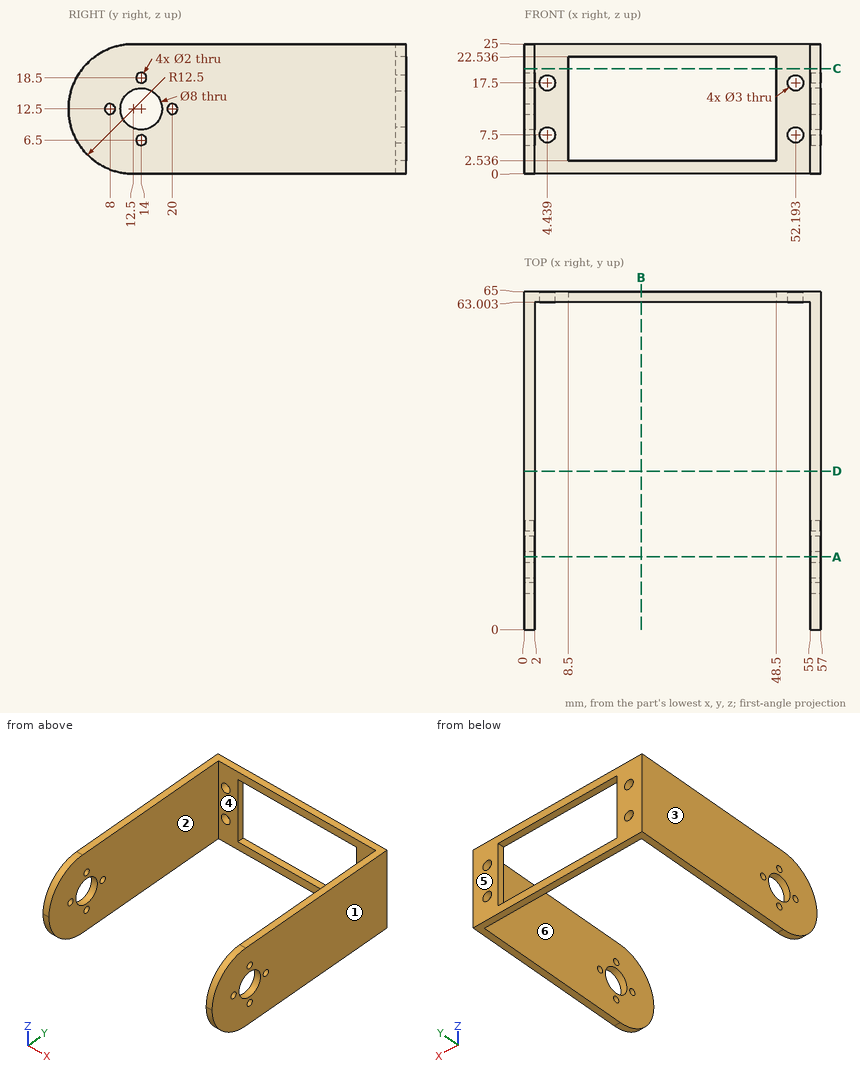
Drawing for the job (mm, zero at the part's lowest x, y, z). A direction names the side the tool comes from. Give positions to 0.01 mm unless a question says otherwise; leave off trailing zeros. Order: outer loops, then holes, each group sorted by start corner. A loop starts at its lowest first (then second) coordinate and runs counter-clockwise, first axis right, second up. Notation, with made-up numbers: M 59,29.25 L 70,29.25 A16 cw 70,41.25 Z; hole C 38.25,-37 d6. An arc over 180 degrees is marked long. Write item = value, one per line. Start each with the question number.
(1) Slice it at C-C on z = 20.25. Write the cut outline in (x, y), plus the area to 3 significant figures.
(2) Probe L1, parallel to X at y = 63.8, z = 17.5; L2, parallel to Z at x = 1.55, y = 14; L3, parallel to X at y = 36, z = 9.75. List the from-to ranges inside material, lowest first. Write a range as [from, to].
(3) Slice it at A-A on y = 14. State how many separate pieces and enclosed holes the cut face has.
(4) Slice it at D-D on y = 30.5. Write the cut outline in (x, z), plus the area to 3 significant figures.
(5) Slice it at B-B on x = 22.5. Write the cut outline in (y, z) (1 decimal).
(6) Two-plate mould, pull along X, no slides. Class the marked faces 3, 4, 5 and 6: released by +X, released by -X, zero draft, split by the parting line, or undercut.
(7) Which spindle directions (+Z, -Z, +X, -X, +Y, -Y) get a long thin tool onto all of the face, cutting with end or side? Do the marked faces 1 and 2. Say none if no direction does.
Responses:
q1.outline = M 0,2.69 L 2,2.69 L 2,63 L 8.5,63 L 8.5,65 L 0,65 Z; M 48.5,63 L 55,63 L 55,2.69 L 57,2.69 L 57,65 L 48.5,65 Z
q1.area = 275 mm2
q2.L1 = [0, 2.94], [5.94, 8.5], [48.5, 50.69], [53.69, 57]
q2.L2 = [0, 5.5], [7.5, 8.5], [16.5, 17.5], [19.5, 25]
q2.L3 = [0, 2], [55, 57]
q3.separate_pieces = 8
q3.enclosed_holes = 0
q4.outline = M 0,0 L 2,0 L 2,25 L 0,25 Z; M 55,0 L 57,0 L 57,25 L 55,25 Z
q4.area = 100 mm2
q5.outline = M 63,0 L 65,0 L 65,2.5 L 63,2.5 Z; M 63,22.5 L 65,22.5 L 65,25 L 63,25 Z
q6.face_3 = released by -X
q6.face_4 = undercut
q6.face_5 = zero draft
q6.face_6 = undercut
q7.face_1 = +Z, -Z, +X, +Y, -Y
q7.face_2 = +Z, -Z, -Y
